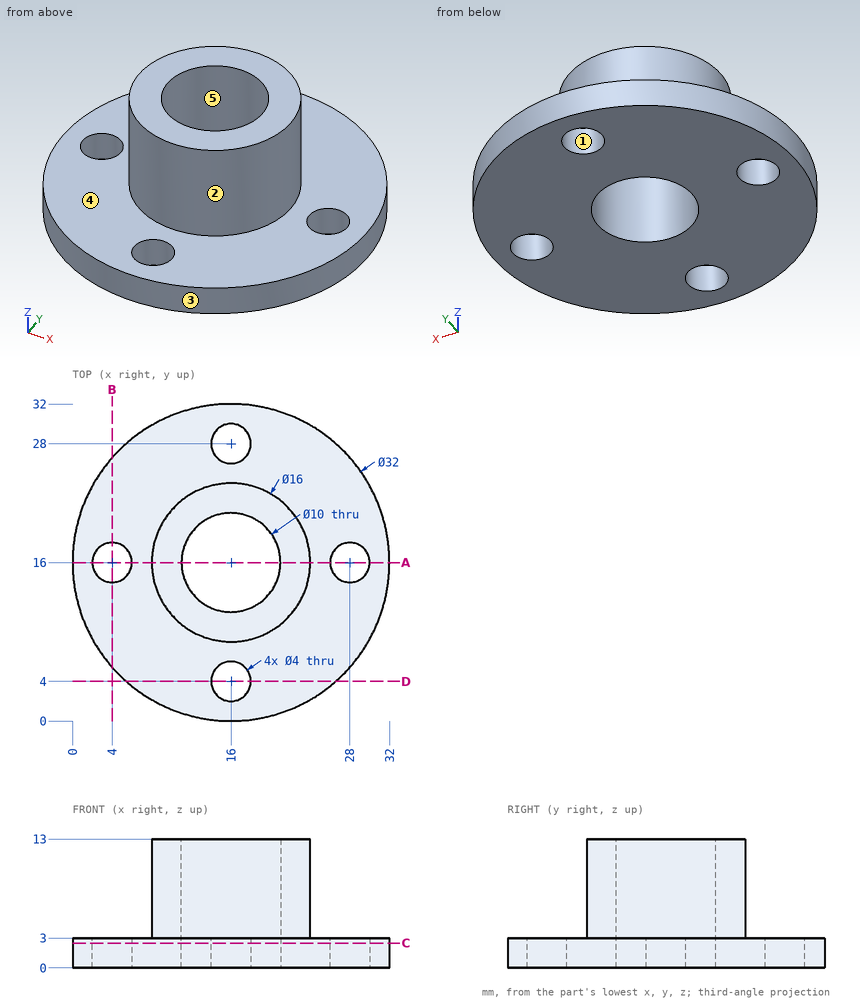
Can you work these out from the drawing? Everything is in mm from the part's minimum corner. A direction names the side the tool comes from. Round coordinates to 2 decimals unless told otherwise and drop trailing zeros. Write each loop counter-clockwise with the first axis right and the second up, starting at its lowest first coordinate (ties: lowest second). Pieces come first, ordered by that corner, then holes. Notation, with made-up numbers: (46.25, -15.75) - (50.25, -15.75) arc R30 cw to (50.25, 22.25) - close; hole circle Ø1 at (60.5, -9.5). An arc over 180 degrees is marked (long way). Put each result on its own line as item: value. Start each with the question number.
(1) I need wall thicknesses on probe 1 along Y at (x, z) = (16, 1.55); probe 2 along Y at (x, z) = (16, 6.5); probe 3 along Z at (x, y) = (31, 19). Which ranges of each line are inside material? Lowest first, please.
(2) I want a section at B-B, the plane x = 4. Please give me the cut outline in (y, z), plus the area to 3 significant figures.
(3) Will these pins go through, and if not, where does the flat tip stop? pin 1 (5 mm diameter, centred on x = 4.5, z = 2.5, fed in from +Y); pin 2 (5 mm diameter, centred on x = 28, y = 16, fed in from -Z); pin 3 (6 mm diameter, centred on y = 19.5, z = 9.5, fed in from +X); pin 4 (2 mm diameter, centred on x = 10.5, z = 1.5, fed in from +Y).
(4) For the marked faces 1 and 2, which set-ups out of +Z, -Z, +X, -X, +Y, -Y let a thin tool reach every point of the face, with its end or its side?
(5) I want a section at A-A, the plane y = 16. Please give me the cut outline in (x, z).
(6) I want a section at C-C, the plane z = 2.5. Please give me the cut outline in (x, y).
(7) Thinking about a two-plate mould opening in Y: for the marked faces 3, 4 and 5, which applies, released by +Y, released by -Y, zero draft, split by the parting line, or undercut?
Here are the results:
1. probe 1: y = 0 to 2, 6 to 11, 21 to 26, 30 to 32
1. probe 2: y = 8 to 11, 21 to 24
1. probe 3: z = 0 to 3
2. outline: (5.42, 0) - (14, 0) - (14, 3) - (5.42, 3) - close; (18, 0) - (26.58, 0) - (26.58, 3) - (18, 3) - close
2. area: 51.5 mm^2
3. pin 1: stops at y = 29.23
3. pin 2: stops at z = 0
3. pin 3: stops at x = 23.98
3. pin 4: stops at y = 31.35
4. face 1: +Z, -Z
4. face 2: +Z
5. outline: (0, 0) - (2, 0) - (2, 3) - (0, 3) - close; (6, 0) - (11, 0) - (11, 13) - (8, 13) - (8, 3) - (6, 3) - close; (21, 0) - (26, 0) - (26, 3) - (24, 3) - (24, 13) - (21, 13) - close; (30, 0) - (32, 0) - (32, 3) - (30, 3) - close
6. outline: circle Ø32 at (16, 16); hole circle Ø4 at (4, 16); hole circle Ø10 at (16, 16); hole circle Ø4 at (16, 4); hole circle Ø4 at (16, 28); hole circle Ø4 at (28, 16)
7. face 3: split by the parting line
7. face 4: zero draft
7. face 5: undercut
